Build history of the part. All positions in model axes, mm. Round coordinates to 2 decimals unless told otherwise and drop trailing zeros. Write each loop counter-clockwise with the first axis right and the second up, starting at its lowest first coordinate (ties: lowest second). Pieces come first, ordered by that corner, then holes. Notation, with made-up numbers: (67.25, 46.25) -> (87.25, 46.25) arc R20 cw to (87.25, 61.25) -> close; hole circle Ø5 at (16.5, 68.25). An arc over 180 degrees is marked (long way). Return JSON: item names as keys, results as strings.
Autodesk Inventor part; units mm, degrees
ref_plane "YZ Plane" through (0, 0, 0) normal (1, 0, 0) x (0, 1, 0)
ref_plane "XZ Plane" through (0, 0, 0) normal (0, 1, 0) x (-1, 0, 0)
ref_plane "XY Plane" through (0, 0, 0) normal (0, 0, 1) x (1, 0, 0)
sketch "Sketch1" plane through (0, 0, 0) normal (0, 0, 1) x (1, 0, 0)
  circle A0 centre (0, 0) radius 67
  circle A1 centre (0, 0) radius 250
  dimension "d0" = 134
  dimension "d1" = 500
extrude "Extrusion1" add sketch "Sketch1" along normal blind 10
sketch "Sketch2" plane through (0, 0, 10) normal (0, 0, 1) x (1, 0, 0)
  circle A0 centre (0, 0) radius 225 construction
  circle A1 centre (0, 0) radius 250
  point P0 (0, 225)
  dimension "d4" = 450
hole "Hole1" at (0, 225, 10) direction (0, 0, -1) diameter 9 end through all
pattern_circular "Circular Pattern1" count 16 over 360 about axis through (0, 0, 0) along (0, 0, 1) of "Hole1"
sketch "Sketch3" plane through (0, 0, 10) normal (0, 0, 1) x (1, 0, 0)
  circle A0 centre (0, 0) radius 170 construction
  point P0 (0, 170)
  dimension "d16" = 340
hole "Hole2" at (0, 170, 10) direction (0, 0, -1) diameter 13 end through all
pattern_circular "Circular Pattern2" count 8 over 360 about axis through (0, 0, -10) along (0, 0, 1) of "Hole2"
equation "\"d22\" = Thickness"
equation "\"BendRadius\" = Thickness"
equation "\"BendReliefWidth\" = Thickness"
equation "\"BendReliefDepth\" = 0.5 * Thickness"
equation "\"CornerReliefSize\" = 4 * Thickness"
equation "\"MinimumRemnant\" = 2 * Thickness"
equation "\"TransitionRadius\" = BendRadius"
equation "\"JacobiRadiusSize\" = BendRadius"
equation "\"GapSize\" = Thickness"
properties part number "DMF pancake"
Q1. Saw through at B-B on x = 42. List the corners of the cut face in (y, z).
Verdict:
{"outline": "(-246.45, 0) -> (-52.2, 0) -> (-52.2, 10) -> (-246.45, 10) -> close; (52.2, 0) -> (246.45, 0) -> (246.45, 10) -> (52.2, 10) -> close"}
Q2. Two-plate mould, pull along Y, no slides. Class faces 1 (the flat face through (52, -52, 10)), 2 (the cylindrical face through (-113.86, -121.61, 4.93)), 3 (the cylindrical face through (-249.76, -10.99, 4.93)): +Y half, -Y half, draft (parallel to the pull), parting line (faces both ways), or undercut.
Verdict:
{"face 1": "draft", "face 2": "undercut", "face 3": "parting line"}
Q3. Pin check, flat tips, straight feed: pin 1 Ø11.5 at (x, y) = (120.21, -120.21) entering from +Z; pin 2 Ø1.5 at (x, z) = (154.5, 5.5) entering from +Y; pin 3 Ø5 at (y, z) = (133, 8) entering from +X; pin 4 Ø2 at (x, z) = (-134.5, 3.5) entering from -Y. Stop position of each tip, or through.
Verdict:
{"pin 1": "passes through", "pin 2": "stops at y = 197.13", "pin 3": "stops at x = 213.24", "pin 4": "stops at y = -211.37"}
Q4. Saw through at A-A on y = 170. List the corners of the cut face in (x, z), then the cut area to 3 significant figures.
Verdict:
{"outline": "(-183.3, 0) -> (-6.5, 0) -> (-6.5, 10) -> (-183.3, 10) -> close; (6.5, 0) -> (183.3, 0) -> (183.3, 10) -> (6.5, 10) -> close", "area": "3,540 mm²"}
Q5. Saw through at D-D on y = -147. List the corners of the cut face in (x, z).
Verdict:
{"outline": "(-202.22, 0) -> (202.22, 0) -> (202.22, 10) -> (-202.22, 10) -> close"}
Q6. Wall check: L1, parallel to X at y = -210, z = 6.75; L2, parallel to X at y = 6, z = 5; L3, parallel to Y at x = -99, z = 2.5. Give the ranges that are in metal, low to high.
Verdict:
{"L1": "x = -135.65 to -90.07, -82.14 to 82.14, 90.07 to 135.65", "L2": "x = -249.93 to -172.5, -167.5 to -66.73, 66.73 to 167.5, 172.5 to 249.93", "L3": "y = -229.56 to 229.56"}
